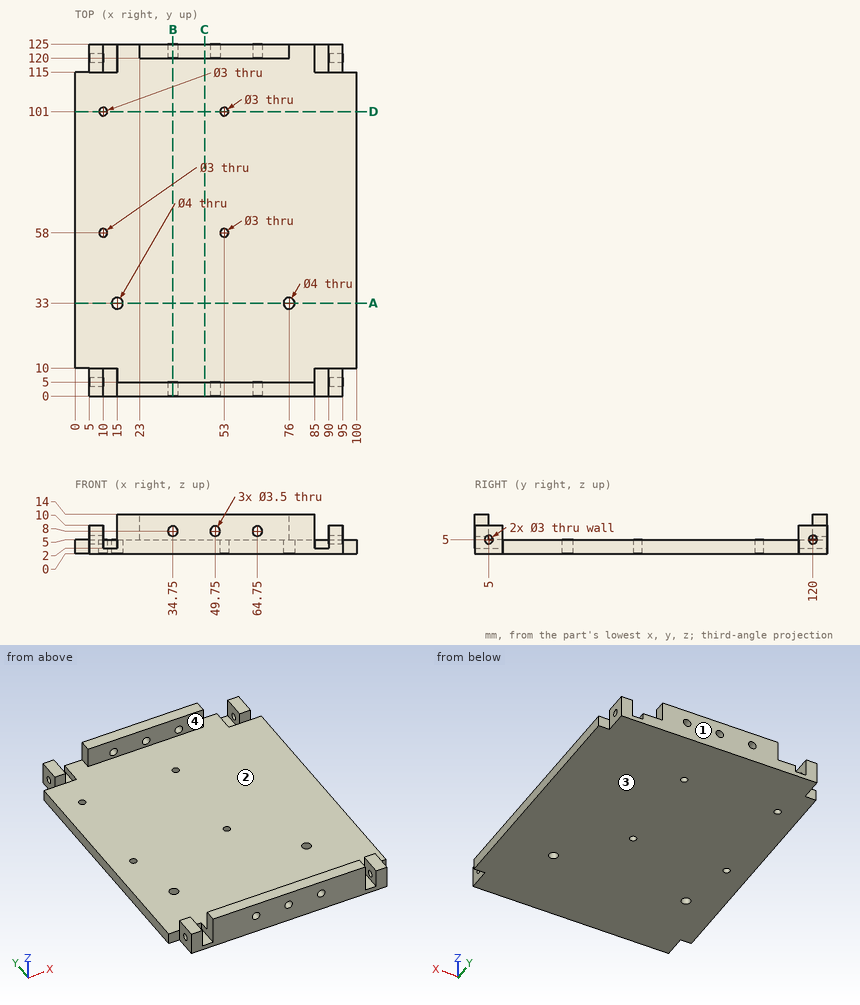
Study the drawing (mm; zero at the part's minimum x, y, z) and answer. Round coordinates to 2 decimals unless told otherwise and drop trailing zeros. Order: outer loops, then holes, each group sorted by start corner. A loop starts at its lowest first (then second) coordinate and runs counter-clockwise, first axis right, second up. Notation, with made-up numbers: M -16,-2 L 32,-2 A7 cw 32,9 Z; hole C 86.25,59 d5. An arc over 180 degrees is marked long. One line per item, written item: value.
Q1. Flat-ended cylindrical pins translate along their axes: pin 1 (6 mm diameter, centred on y = 106.5, z = 9, fed in from -X); pin 2 (0.9 mm diameter, centred on y = 118.5, z = 3.5, fed in from -X); pin 3 (5.5 mm diameter, centred on x = 8.5, y = 122, fed in from +Z); pin 4 (5 mm diameter, centred on x = 10, y = 101, fed in from +Z). Find the tip coordinate at first contact, or state that the pin passes through.
Derived:
pin 1: through
pin 2: x = 5
pin 3: z = 10
pin 4: z = 5
Q2. Find section D-D on y = 101. Write down the section's boundary in (x, z), then the cut area to 3 significant figures.
Derived:
outline: M 0,0 L 8.5,0 L 8.5,5 L 0,5 Z; M 11.5,0 L 51.5,0 L 51.5,5 L 11.5,5 Z; M 54.5,0 L 100,0 L 100,5 L 54.5,5 Z
area: 470 mm²
Q3. Find section A-A on y = 33. Write down the section's boundary in (x, z), then the cut area to 3 significant figures.
Derived:
outline: M 0,0 L 13,0 L 13,5 L 0,5 Z; M 17,0 L 74,0 L 74,5 L 17,5 Z; M 78,0 L 100,0 L 100,5 L 78,5 Z
area: 460 mm²
Q4. Find section C-C on x = 46. Write down the section's boundary in (y, z), then the cut area to 3 significant figures.
Derived:
outline: M 0,0 L 125,0 L 125,14 L 120,14 L 120,5 L 5,5 L 5,14 L 0,14 Z
area: 715 mm²
Q5. Determine the mould class of the marked faces 1, 2, 3 and 4 for opening direction Y: released by +Y, released by -Y, zero draft, split by the parting line, or undercut.
Derived:
face 1: released by +Y
face 2: undercut
face 3: zero draft
face 4: undercut
Q6. Straight lines are drawn through the part: line 1 (X direction, y = 101, z = 2.5); line 2 (Y direction, x = 47, z = 10.5); line 3 (X direction, y = 3.3, z = 8). For each, find the intervals that lie inside material, in ascending order.
Derived:
line 1: 0 to 8.5, 11.5 to 51.5, 54.5 to 100
line 2: 0 to 5, 120 to 125
line 3: 5 to 10, 15 to 33, 36.5 to 48, 51.5 to 63, 66.5 to 85, 90 to 95
Q7. Find section B-B on x = 34.75. Write down the section's boundary in (y, z), then the cut area to 3 significant figures.
Derived:
outline: M 0,0 L 125,0 L 125,6.25 L 120,6.25 L 120,5 L 5,5 L 5,6.25 L 0,6.25 Z; M 0,9.75 L 5,9.75 L 5,14 L 0,14 Z; M 120,9.75 L 125,9.75 L 125,14 L 120,14 Z
area: 680 mm²
